Build history of the part. All positions in model axes, mm. Face numbers are marked on the shaded views. A direction names the side the tool comes from. Round coordinates to 2 decimals unless told otherwise and drop trailing zeros. Loops run counter-clockwise (first coordinate to the right, second up) from the corner with the lowest first, then second, coordinate; pieces in that order, holes last. Notation, with made-up numbers: (39.5, 56.25) - (71.5, 56.25) arc R22 cw to (71.5, 78.25) - close; hole circle Ø10 at (46, 13.25). An arc over 180 degrees is marked (long way). One line per question, with ' | ' between items. Start each with the question number.
from build123d import *

# Parameters (mm, degrees)
SKETCH1_W           = 98
SKETCH1_H           = 25
BOSS_EXTRUDE1_DEPTH = 10
SKETCH4_W           = 25
SKETCH4_H           = 10
CUT_EXTRUDE6_DEPTH  = 5
SKETCH5_W           = 25
SKETCH5_H           = 10
CUT_EXTRUDE7_DEPTH  = 5
SKETCH6_W           = 5
SKETCH6_H           = 10
CUT_EXTRUDE8_DEPTH  = 5
SKETCH7_W           = 5
SKETCH7_H           = 10
CUT_EXTRUDE9_DEPTH  = 5
SKETCH8_W           = 50
SKETCH8_H           = 20.9
CUT_EXTRUDE10_DEPTH = 13
SKETCH9_W           = 15.1
SKETCH9_H           = 7.5
SKETCH9_H_2         = 12.5
CUT_EXTRUDE11_DEPTH = 13
SKETCH10_W          = 15.1
SKETCH10_H          = 5
CUT_EXTRUDE12_DEPTH = 3.3


with BuildPart() as part:
    # Sketch1 → Boss-Extrude1 (new body)
    with BuildSketch(Plane(origin=(0, 0, 0), x_dir=(1, 0, 0), z_dir=(0, 1, 0))):
        Rectangle(SKETCH1_W, SKETCH1_H)
    extrude(amount=BOSS_EXTRUDE1_DEPTH)

    # Sketch4 → Cut-Extrude6 (cut)
    with BuildSketch(Plane.ZY.offset(49)):
        with Locations((0, 5)):
            Rectangle(SKETCH4_W, SKETCH4_H)
    extrude(amount=-CUT_EXTRUDE6_DEPTH, mode=Mode.SUBTRACT)

    # Sketch5 → Cut-Extrude7 (cut)
    with BuildSketch(Plane(origin=(49, 0, 0), x_dir=(0, 0, -1), z_dir=(1, 0, 0))):
        with Locations((0, 5)):
            Rectangle(SKETCH5_W, SKETCH5_H)
    extrude(amount=-CUT_EXTRUDE7_DEPTH, mode=Mode.SUBTRACT)

    # Sketch6 → Cut-Extrude8 (cut)
    with BuildSketch(Plane(origin=(44, 0, 0), x_dir=(0, 0, -1), z_dir=(1, 0, 0))):
        with Locations((0, 5)):
            Rectangle(SKETCH6_W, SKETCH6_H)
    extrude(amount=-CUT_EXTRUDE8_DEPTH, mode=Mode.SUBTRACT)

    # Sketch7 → Cut-Extrude9 (cut)
    with BuildSketch(Plane.ZY.offset(44)):
        with Locations((0, 5)):
            Rectangle(SKETCH7_W, SKETCH7_H)
    extrude(amount=-CUT_EXTRUDE9_DEPTH, mode=Mode.SUBTRACT)

    # Sketch8 → Cut-Extrude10 (cut)
    with BuildSketch(Plane(origin=(0, 10, 0), x_dir=(1, 0, 0), z_dir=(0, 1, 0))):
        with Locations((9, -2.05)):
            Rectangle(SKETCH8_W, SKETCH8_H)
    extrude(amount=-CUT_EXTRUDE10_DEPTH, mode=Mode.SUBTRACT)

    # Sketch9 → Cut-Extrude11 (cut)
    with BuildSketch(Plane(origin=(0, 10, 0), x_dir=(1, 0, 0), z_dir=(0, 1, 0))):
        with Locations((-27.5, 3.75)):
            Rectangle(SKETCH9_W, SKETCH9_H)
        with Locations((-27.5, -6.25)):
            Rectangle(SKETCH9_W, SKETCH9_H_2)
    extrude(amount=-CUT_EXTRUDE11_DEPTH, mode=Mode.SUBTRACT)

    # Sketch10 → Cut-Extrude12 (cut)
    with BuildSketch(Plane.XZ):
        with Locations((-27.5, -10)):
            Rectangle(SKETCH10_W, SKETCH10_H)
    extrude(amount=-CUT_EXTRUDE12_DEPTH, mode=Mode.SUBTRACT)


solid = part.part
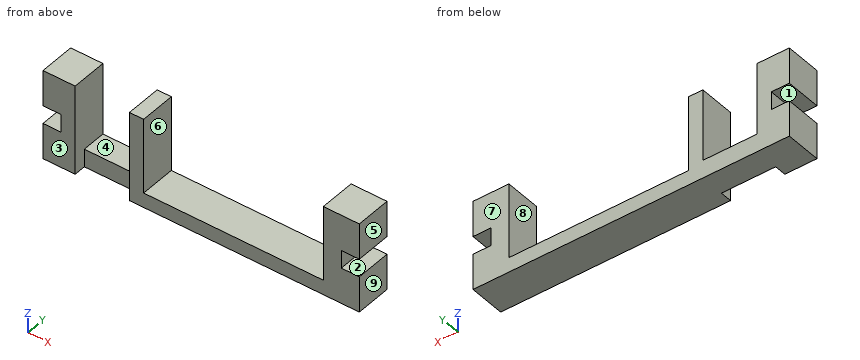
1) Saw through at A-A on z = 0. Write the cut outline in (x, y), and give its area (3 significant figures).
2) Two-plate mould, pull along X, no slides. Class the marked faces 6, 7, 8 and 9: +X half, -X half, draft (parallel to the pull), parting line (faces both ways), or undercut.
3) Wall check: line 1 (X direction, y = 7.75, z = 2.25); line 2 (X direction, y = 6.25, z = 9.5); line 3 (X direction, y = 3.5, z = -7.75). Give the ranges that are in metal, low to high. Write a range as [from, to].
4) Saw through at D-D on z = 4.5. Write the cut outline in (x, y).
5) Saw through at C-C on y = 6.25. Write the cut outline in (x, z), and give its area (3 significant figures).
6) Tool access for the marked faces 1, 2, 3, 4 and 5: list every direction of +Z, -Z, +X, -X, +Y, -Y with a clear straight run to the whole face (end or side of a thin tool).
7) Drop flat-ended pins along their axis: pin 1 (5 mm diameter, centred on y = 4.5, z = 2, fed in from +X); pin 2 (5 mm diameter, centred on x = -27, y = 2, fed in from +Z); pin 3 (5 mm diameter, centred on x = -30, z = -7.5, fed in from -Y). Give the stop position or say it passes through.
8) Saw through at B-B on y = 1.5. Write the cut outline in (x, z).
Answer key:
1) outline: (-39, 0) - (-35.05, 0) - (-35.05, 10) - (-39, 10) - close; (-19.95, 0) - (-16, 0) - (-16, 10) - (-19.95, 10) - close; (34, 0) - (39, 0) - (39, 10) - (34, 10) - close | area: 129 mm²
2) face 6: undercut | face 7: draft | face 8: undercut | face 9: +X half
3) line 1: [-39, -35.05], [-19.95, -16], [34, 39] | line 2: [-44, -35.05], [-19.95, -16], [34, 44] | line 3: [-44, -16], [34, 44]
4) outline: (-44, 0) - (-35.05, 0) - (-35.05, 10) - (-44, 10) - close; (-19.95, 0) - (-16, 0) - (-16, 10) - (-19.95, 10) - close; (34, 0) - (44, 0) - (44, 10) - (34, 10) - close
5) outline: (-44, -12.5) - (44, -12.5) - (44, -2.5) - (39, -2.5) - (39, 2.5) - (44, 2.5) - (44, 12.5) - (34, 12.5) - (34, -8.4) - (-16, -8.4) - (-16, 12.5) - (-19.95, 12.5) - (-19.95, -7.5) - (-35.05, -7.5) - (-35.05, 12.5) - (-44, 12.5) - (-44, 2.5) - (-39, 2.5) - (-39, -2.5) - (-44, -2.5) - close | area: 803 mm²
6) face 1: -X, +Y, -Y | face 2: +X, +Y, -Y | face 3: +Z, -Z, +X, -X, -Y | face 4: +Z, +Y, -Y | face 5: +Z, -Z, +X, +Y, -Y
7) pin 1: x = 44 | pin 2: z = -7.5 | pin 3: y = 3.3
8) outline: (-44, -12.5) - (-35.05, -12.5) - (-35.05, 12.5) - (-44, 12.5) - (-44, 2.5) - (-39, 2.5) - (-39, -2.5) - (-44, -2.5) - close; (-19.95, -12.5) - (44, -12.5) - (44, -2.5) - (39, -2.5) - (39, 2.5) - (44, 2.5) - (44, 12.5) - (34, 12.5) - (34, -8.4) - (-16, -8.4) - (-16, 12.5) - (-19.95, 12.5) - close
